Job drawing, mm, ordinate dimensions from the low corner. One solid piece. Give positions to 0.01 mm unless a question says otherwise; leave off trailing zeros. Loops run counter-clockwise (first coordinate to the right, second up) from the corner with the lowest first, then second, coordinate; pieces in that order, holes last. Notation, with made-up numbers: (80, 76) - (116, 76) arc R32 cw to (116, 107) - close; hole circle Ø11 at (28.25, 21). An arc over 180 degrees is marked (long way). Use a Markdown table: item, result.
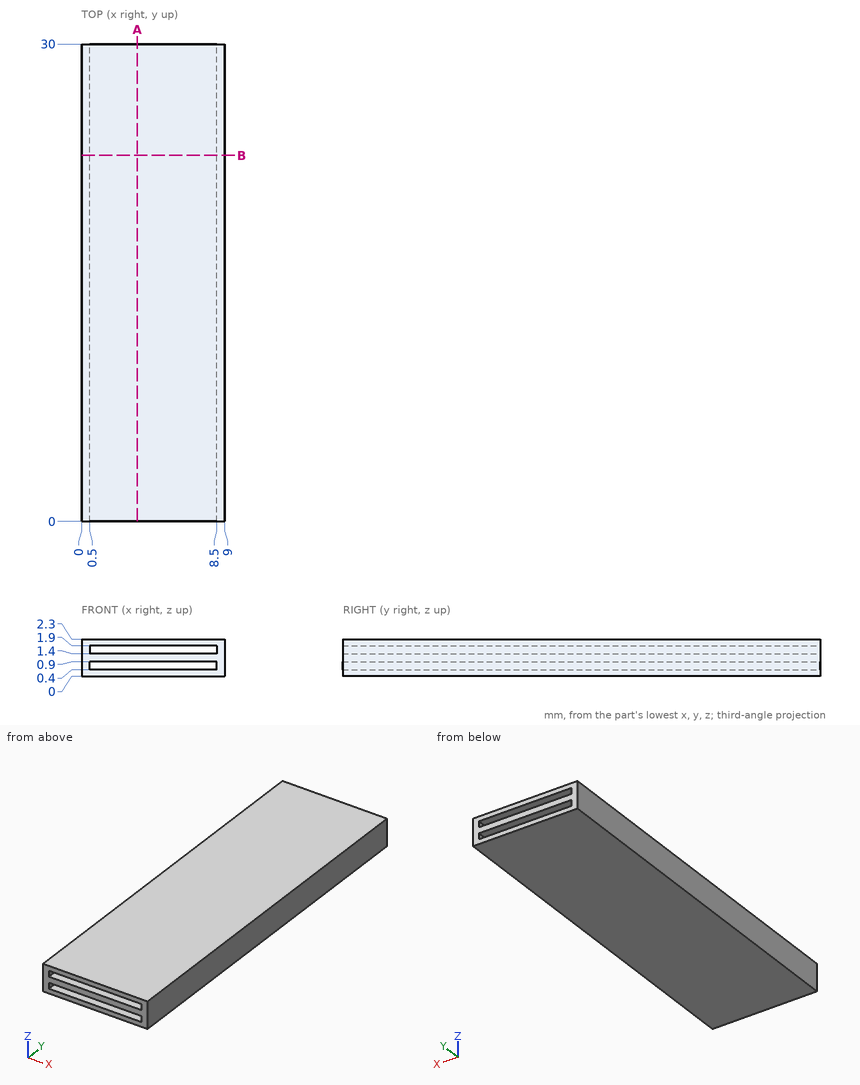
(1) Drill centre lines: probe 1 along Z at (x, y) = (1.25, 17); probe 2 along X at (y, z) = (7.5, 0.6). Where is each one in solid material? Low to high. Write a range as [from, to].
Computed:
| item | result |
|---|---|
| probe 1 | [0, 0.4], [0.9, 1.4], [1.9, 2.3] |
| probe 2 | [0, 0.5], [8.5, 9] |
(2) Slice it at B-B, the plane y = 23. Write the cut outline in (x, z), plus the area to 3 significant figures.
Computed:
| item | result |
|---|---|
| outline | (0, 0) - (9, 0) - (9, 2.3) - (0, 2.3) - close; hole (0.5, 0.4) - (8.5, 0.4) - (8.5, 0.9) - (0.5, 0.9) - close; hole (0.5, 1.4) - (8.5, 1.4) - (8.5, 1.9) - (0.5, 1.9) - close |
| area | 12.7 mm² |
(3) Slice it at A-A, the plane x = 3.5. Write the cut outline in (y, z), plus the area to 3 significant figures.
Computed:
| item | result |
|---|---|
| outline | (0, 0) - (30, 0) - (30, 0.4) - (0, 0.4) - close; (0, 0.9) - (30, 0.9) - (30, 1.4) - (0, 1.4) - close; (0, 1.9) - (30, 1.9) - (30, 2.3) - (0, 2.3) - close |
| area | 39.0 mm² |
